The model under review builds one solid part; all positions refer to its coordinate system, in mm. Face numbers are marked on the shaded views. A direction names the side the tool comes from. Give positions to 0.01 mm unless a question says otherwise; leave off trailing zeros. Loops run counter-clockwise (first coordinate to the right, second up) from the corner with the lowest first, then second, coordinate; pieces in that order, holes last. Notation, with made-up numbers: (30.5, 23) - (44.5, 23) arc R26 ccw to (44.5, 42) - close; hole circle Ø8 at (-23, -30.75). An arc over 180 degrees is marked (long way). Return JSON: item names as keys, results as strings. Group by question number.
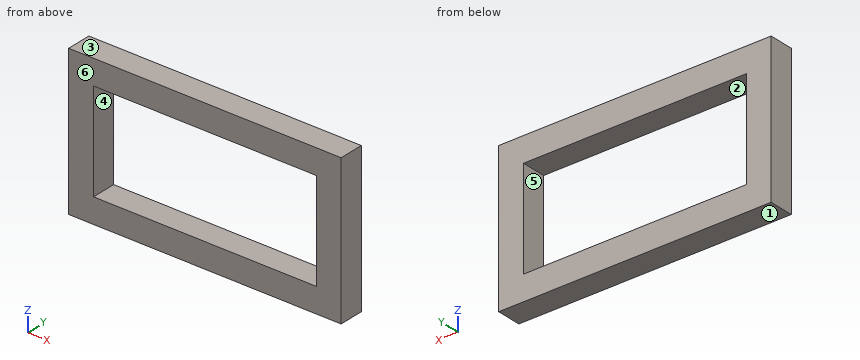
```python
from build123d import *

# Parameters (mm, degrees)
SKETCH_1_W      = 180
SKETCH_1_H      = 80
EXTRUDE_1_DEPTH = 20


with BuildPart() as part:
    # 草图1 → 凸台-拉伸1 (new body)
    with BuildSketch(Plane(origin=(0, 0, 0), x_dir=(1, 0, 0), z_dir=(0, 1, 0))):
        Polygon((-110, -40), (-110, -60), (110, -60), (110, -40), (110, 40), (110, 59.931716483), (-110, 59.931716483), (-110, 40), align=None)
        Rectangle(SKETCH_1_W, SKETCH_1_H, mode=Mode.SUBTRACT)
    extrude(amount=-EXTRUDE_1_DEPTH)


solid = part.part
```
1) We need section B-B, the plane x = 70.5. Write out the cut boundary in (y, z).
2) We need section C-C, the plane y = -12.75. Write out the cut boundary in (x, z), plus the area to 3 significant figures.
3) To check wall thickness, follow line 1 (Z direction, x = 77.5, y = -1.75); line 2 (X direction, y = -11.75, z = 26). State the ranges of each line that lie inside material, in increasing order.
4) We need section A-A, the plane z = -8.5. Write out the cut boundary in (x, y), plus the area to 3 significant figures.
5) Draft analysis for pull direction Z (two halves, no side actions). For the marked faces 1, 2, 3 and 4, state which applies: +Z half, -Z half, draft (parallel to the pull), parting line (faces both ways), or undercut.
6) Tool access review of the marked faces 5 and 6: name each direction out of +Z, -Z, +X, -X, +Y, -Y from which nothing blocks a thin tool from reaching the whole face with its end or side.
Findings:
{
 "1": {"outline": "(-20, -59.93) - (0, -59.93) - (0, -40) - (-20, -40) - close; (-20, 40) - (0, 40) - (0, 60) - (-20, 60) - close"},
 "2": {"outline": "(-110, -59.93) - (110, -59.93) - (110, 60) - (-110, 60) - close; hole (-90, -40) - (90, -40) - (90, 40) - (-90, 40) - close", "area": "12,000 mm^2"},
 "3": {"line 1": "z = -59.93 to -40, 40 to 60", "line 2": "x = -110 to -90, 90 to 110"},
 "4": {"outline": "(-110, -20) - (-90, -20) - (-90, 0) - (-110, 0) - close; (90, -20) - (110, -20) - (110, 0) - (90, 0) - close", "area": "800 mm^2"},
 "5": {"face 1": "-Z half", "face 2": "undercut", "face 3": "+Z half", "face 4": "undercut"},
 "6": {"face 5": "+Y, -Y", "face 6": "+Z, -Z, +X, -X, -Y"}
}
